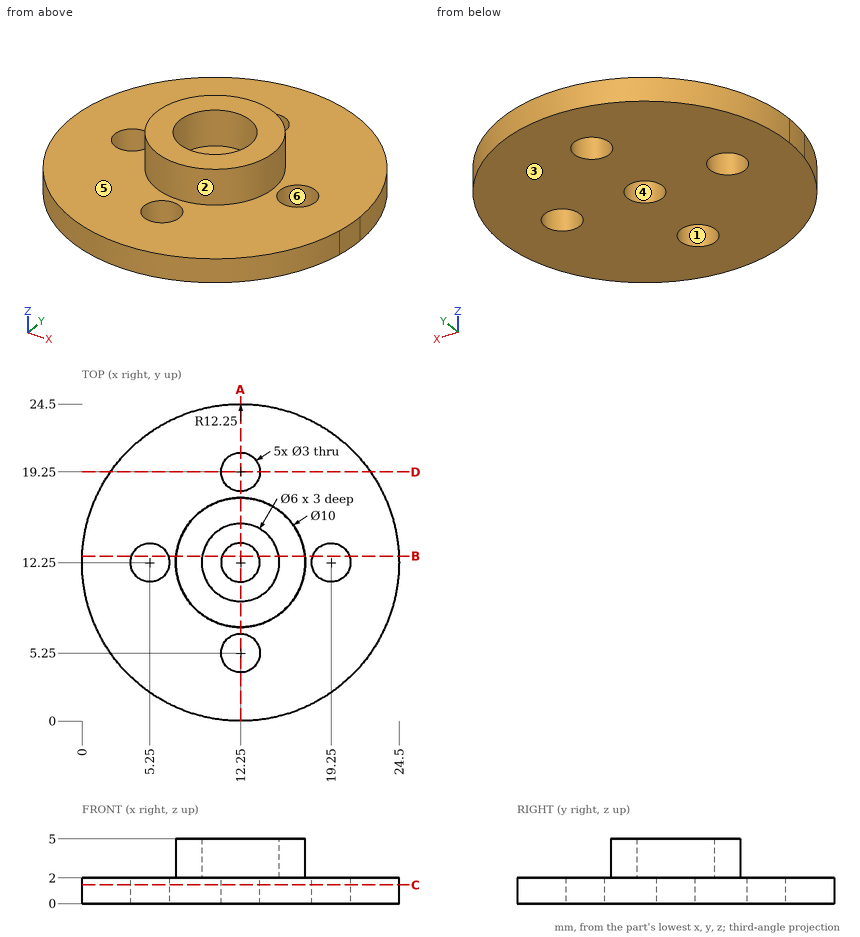
Could you check a few things on this drawing? It's one solid part, dimensions in mm from its lowest x, y, z. A direction names the side the tool comes from. Give positions to 0.01 mm unless a question says otherwise; leave off trailing zeros. Order: outer loops, then holes, each group sorted by start corner. A loop starts at its lowest first (then second) coordinate and runs counter-clockwise, first axis right, second up. Notation, with made-up numbers: (5, 37) - (55, 37) arc R24 cw to (55, 63) - close; hole circle Ø5 at (-18.5, -25). An arc over 180 degrees is marked (long way). Answer as a JSON object with one key per item and string values. Group by question number.
Item 1: If we section it at D-D on y = 19.25: Please give me the cut outline in (x, z).
Item 2: If we section it at A-A on x = 12.25: Please give me the cut outline in (y, z), and give its area (3 significant figures).
Item 3: If we mould it in two halves opening along X, with no side actions, what happens to the marked faces 1, 2, 3 and 4? For each: pulls with the +X half, pulls with the -X half, needs draft (parallel to the pull), parting line crosses it, or undercut.
Item 4: Which directions (+Z, -Z, +X, -X, +Y, -Y) give clear straight access to the entire face, cutting with the end or side of a thin tool? Please do the marked faces 5 and 6.
Item 5: Please list where these lines run through material, in increasing order: probe 1 along Y at (x, z) = (12.25, 1.6); probe 2 along Z at (x, y) = (21, 7.5); probe 3 along X at (y, z) = (10.75, 3.7).
Item 6: If we section it at B-B on y = 12.75: Please give me the cut outline in (x, z).
Item 7: For P1, Ø2.5, axis at x = 12.25, y = 19.25, coming from the +Z side; P2, Ø8, axis at x = 20, y = 3, coming from the +Z side; P3, Ø1.5, axis at y = 17, z = 3, coming from the -X side; P4, Ø1.5, axis at x = 14, z = 0.5, coming from the +Y side, each with a flat end and sliding along its axis, tell me the tip position at first contact or that it passes through.
Item 8: If we section it at C-C on z = 1.45: Please give me the cut outline in (x, y).
Result set:
{
 "1": {"outline": "(2.2, 0) - (10.75, 0) - (10.75, 2) - (2.2, 2) - close; (13.75, 0) - (22.3, 0) - (22.3, 2) - (13.75, 2) - close"},
 "2": {"outline": "(0, 0) - (3.75, 0) - (3.75, 2) - (0, 2) - close; (6.75, 0) - (10.75, 0) - (10.75, 2) - (9.25, 2) - (9.25, 5) - (7.25, 5) - (7.25, 2) - (6.75, 2) - close; (13.75, 0) - (17.75, 0) - (17.75, 2) - (17.25, 2) - (17.25, 5) - (15.25, 5) - (15.25, 2) - (13.75, 2) - close; (20.75, 0) - (24.5, 0) - (24.5, 2) - (20.75, 2) - close", "area": "43.0 mm²"},
 "3": {"face 1": "undercut", "face 2": "parting line crosses it", "face 3": "needs draft", "face 4": "undercut"},
 "4": {"face 5": "+Z", "face 6": "+Z, -Z"},
 "5": {"probe 1": "0 to 3.75, 6.75 to 10.75, 13.75 to 17.75, 20.75 to 24.5", "probe 2": "0 to 2", "probe 3": "7.48 to 9.65, 14.85 to 17.02"},
 "6": {"outline": "(0.01, 0) - (3.84, 0) - (3.84, 2) - (0.01, 2) - close; (6.66, 0) - (10.84, 0) - (10.84, 2) - (9.29, 2) - (9.29, 5) - (7.28, 5) - (7.28, 2) - (6.66, 2) - close; (13.66, 0) - (17.84, 0) - (17.84, 2) - (17.22, 2) - (17.22, 5) - (15.21, 5) - (15.21, 2) - (13.66, 2) - close; (20.66, 0) - (24.49, 0) - (24.49, 2) - (20.66, 2) - close"},
 "7": {"P1": "through", "P2": "z = 2", "P3": "x = 9.25", "P4": "y = 24.46"},
 "8": {"outline": "circle Ø24.5 at (12.25, 12.25); hole circle Ø3 at (5.25, 12.25); hole circle Ø3 at (12.25, 5.25); hole circle Ø3 at (12.25, 12.25); hole circle Ø3 at (12.25, 19.25); hole circle Ø3 at (19.25, 12.25)"}
}
